Geometry check sheet. Reference: the model listing, model coordinates, mm. A direction names the side the tool comes from. Coordinates: 2 decimals unless noted, no trailing zeros. Order: outer loops, then holes, each group sorted by start corner. A loop starts at its lowest first (then second) coordinate and runs counter-clockwise, first axis right, second up. Notation, with made-up numbers: (78, 47) - (98, 47) arc R26 ccw to (98, 79) - close; hole circle Ø2 at (-21, 19.5). An arc over 180 degrees is marked (long way). Put each result on its own line as item: value.
from build123d import *

# Parameters (mm, degrees)
F1_DEPTH = 25.4
F2_W     = 83.970894
F2_H     = 25.4
F3_DEPTH = 6.35
F4_R     = 9.551083
F5_DEPTH = 31.75


with BuildPart() as f1:
    # F0 (on Top) → F1 (new body)
    with BuildSketch(Plane.XY):
        Polygon((67.652024, 57.670575), (-67.335151, 57.670575), (67.652024, -26.300319), align=None)
    extrude(amount=F1_DEPTH)

    # F2 (on face) → F3 (join)
    with BuildSketch(Plane.YZ.offset(67.652024)):
        with Locations((15.685128, 12.7)):
            Rectangle(F2_W, F2_H)
    extrude(amount=F3_DEPTH)

    # F4 (on face) → F5 (join)
    with BuildSketch(Plane.YZ.offset(74.002024)):
        with Locations((15.685128, 12.7)):
            Circle(F4_R)
    extrude(amount=F5_DEPTH)


solid = f1.part
Q1. Thickness scan on L1, parallel to Y at x = -45.5, z = 20; L2, parallel to Y at x = -57, z = 1.5; L3, parallel to X at y = 44, z = 22.5. Record the ranges inside material, lowest first. Write a range as [from, to].
Answer block:
L1: y = [44.09, 57.67]
L2: y = [51.24, 57.67]
L3: x = [-45.36, 74]
Q2. Section check D-D on y = -15. Record the boundary of the cut face in (x, z), then the cut area to 3 significant figures.
Answer block:
outline: (49.49, 0) - (74, 0) - (74, 25.4) - (49.49, 25.4) - close
area: 623 mm^2
Q3. Access from +Z, -Z, +X, -X, +Y, -Y to the whole of each face (thin tool, end or side, straight path). Record for faces 1 (the flat face through (34, 24, 25.4)), 2 (the cylindrical face through (89.655, 6.143, 13.12)).
Answer block:
face 1: +Z, +X, -X, +Y, -Y
face 2: +X
Q4. Section check C-C on y = 22. Record the boundary of the cut face in (x, z).
Answer block:
outline: (-9.99, 0) - (74, 0) - (74, 5.53) - (105.75, 5.53) - (105.75, 19.87) - (74, 19.87) - (74, 25.4) - (-9.99, 25.4) - close
Q5. Section check A-A on z = 12.7. Record the boundary of the cut face in (x, y).
Answer block:
outline: (-67.34, 57.67) - (67.65, -26.3) - (74, -26.3) - (74, 6.13) - (105.75, 6.13) - (105.75, 25.24) - (74, 25.24) - (74, 57.67) - close
Q6. Section check B-B on x = 76. Record the boundary of the cut face in (y, z).
Answer block:
outline: circle Ø19.1 at (15.69, 12.7)
Q7. Depth check by flat-ended pin: pin 1 Ø3 at (y, z) = (-15.5, 17.5) entering from +X; pin 2 Ø1.5 at (x, z) = (63, 19.5) entering from -Y; pin 3 Ø12 at (y, z) = (24, 14.5) entering from -X. Enter the tip coordinate at first touch or a pass-through.
Answer block:
pin 1: stops at x = 74
pin 2: stops at y = -23.87
pin 3: stops at x = -22.85
